Check sheet for the drawn part. Datum: minimum x, y, z corner. Units: mm. Give positions to 0.01 mm unless a question says otherwise; leave off trailing zeros. Write each loop counter-clockwise with the first axis right and the second up, starting at its lowest first coordinate (ties: lowest second). Pieces come first, ordered by that corner, then holes.
(1) Cross-section at A-A (z = 5). Record the boundary of the cut face in (x, y).
(2) Cross-section at D-D (x = 17.7). Record the boundary of the cut face in (y, z).
(3) Depth check by flat-ended pin: P1, Ø4, axis at x = 2, z = 9, coming from the +Y side; P2, Ø1.1, axis at y = 0.5, z = 3.5, coming from the -X side. Enter the tip coordinate at first touch or a pass-through.
(4) Cross-section at C-C (y = 0.7). Record the boundary of the cut face in (x, z).
(5) Cross-section at B-B (x = 11.75). Record the boundary of the cut face in (y, z), and give its area (3 significant figures).
(6) Thickness scan on line 1 along X through (y, z) = (0.1, 3.75); line 2 along Z through (x, y) = (13, 0.85); line 3 along Y through (x, z) = (2.5, 3.25). Record the ranges inside material, lowest first.
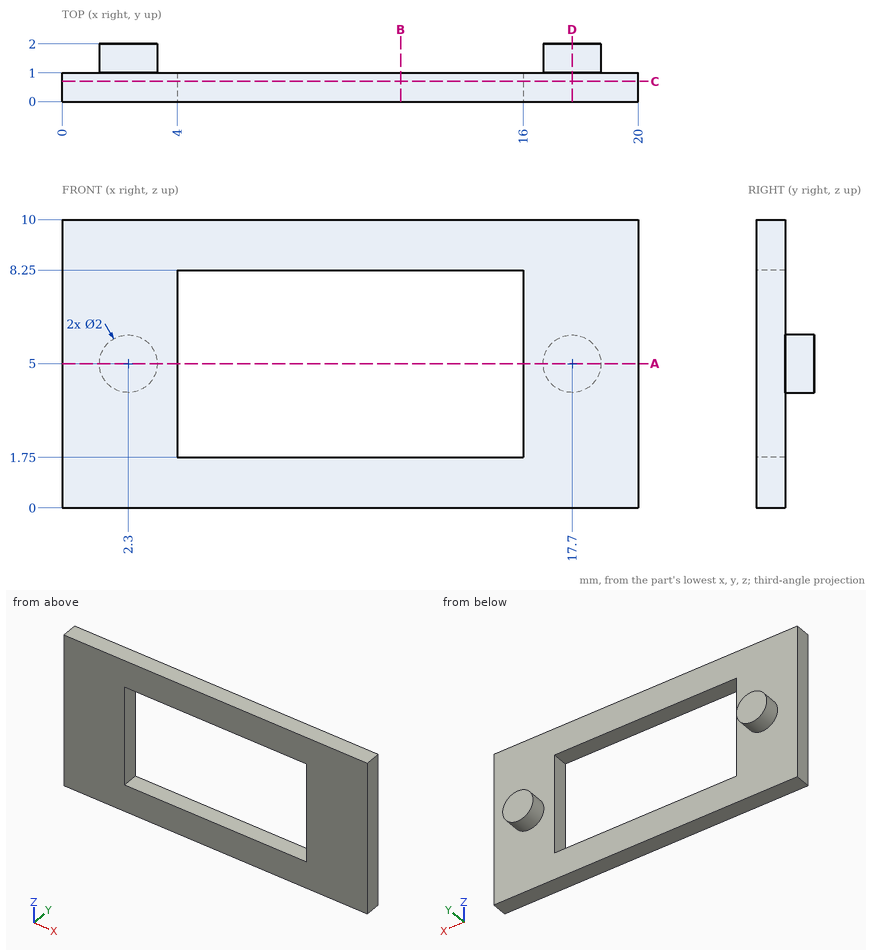
Reply:
1. outline: (0, 0) - (4, 0) - (4, 1) - (3.3, 1) - (3.3, 2) - (1.3, 2) - (1.3, 1) - (0, 1) - close; (16, 0) - (20, 0) - (20, 1) - (18.7, 1) - (18.7, 2) - (16.7, 2) - (16.7, 1) - (16, 1) - close
2. outline: (0, 0) - (1, 0) - (1, 4) - (2, 4) - (2, 6) - (1, 6) - (1, 10) - (0, 10) - close
3. P1: stops at y = 1
3. P2: stops at x = 0
4. outline: (0, 0) - (20, 0) - (20, 10) - (0, 10) - close; hole (4, 1.75) - (16, 1.75) - (16, 8.25) - (4, 8.25) - close
5. outline: (0, 0) - (1, 0) - (1, 1.75) - (0, 1.75) - close; (0, 8.25) - (1, 8.25) - (1, 10) - (0, 10) - close
5. area: 3.50 mm2
6. line 1: x = 0 to 4, 16 to 20
6. line 2: z = 0 to 1.75, 8.25 to 10
6. line 3: y = 0 to 1
